Geometry check sheet. Reference: the model listing, model coordinates, mm. A direction names the side the tool comes from. Give positions to 0.01 mm unless a question says otherwise; leave off trailing zeros. Loops run counter-clockwise (first coordinate to the right, second up) from the corner with the lowest first, then second, coordinate; pieces in that order, holes last. Notation, with made-up numbers: (65, 88.5) -> (96, 88.5) arc R17 cw to (96, 100.5) -> close; hole circle Ø5 at (40, -15.75). An arc over 180 degrees is marked (long way). Answer in a Markdown table with one row per item. Add a question column.
```python
from build123d import *

# Parameters (mm, degrees)
CROQUIS1_W              = 72.136
CROQUIS1_H              = 25.4
SALIENTE_EXTRUIR1_DEPTH = 96.52
VACIADO1_T              = -3
CROQUIS2_W              = 2.032
CROQUIS2_H              = 17.272
SALIENTE_EXTRUIR3_DEPTH = 96.52
CROQUIS4_W              = 16.5
CROQUIS4_H              = 4
SALIENTE_EXTRUIR4_DEPTH = 4.5


with BuildPart() as part:
    # Croquis1 → Saliente-Extruir1 (new body)
    with BuildSketch(Plane.XY):
        with Locations((-36.068, 12.7)):
            Rectangle(CROQUIS1_W, CROQUIS1_H)
    extrude(amount=SALIENTE_EXTRUIR1_DEPTH)

    # Vaciado1
    vaciado1_openings = [part.faces().sort_by_distance(p)[0] for p in [
        (-36.068, 25.4, 48.26),
    ]]
    offset(amount=VACIADO1_T, openings=vaciado1_openings, kind=Kind.INTERSECTION)

    # Croquis2 → Saliente-Extruir3 (add)
    with BuildSketch(Plane(origin=(0, 0, 0), x_dir=(-1, 0, 0), z_dir=(0, 0, -1))):
        with Locations((-1.016, 12.7)):
            Rectangle(CROQUIS2_W, CROQUIS2_H)
        with Locations((73.152, 12.7)):
            Rectangle(CROQUIS2_W, CROQUIS2_H)
    extrude(amount=-SALIENTE_EXTRUIR3_DEPTH)

    # Croquis4 → Saliente-Extruir4 (add)
    with BuildSketch(Plane(origin=(0, 0, 0), x_dir=(-1, 0, 0), z_dir=(0, 0, -1))):
        with Locations((36.068, 3.262624702)):
            Rectangle(CROQUIS4_W, CROQUIS4_H)
    extrude(amount=SALIENTE_EXTRUIR4_DEPTH)


solid = part.part
```
1. Sectioned sample at D-D (y = 22.5). Enter the section's corners in (x, z).
2. Material ranges on L1, parallel to X at y = 11.5, z = 55; L2, parallel to Z at x = -30, y = 12.75; L3, parallel to X at y = 21.75, z = 85, recorded low to high. Write a range as from..to.
3. Sectioned sample at C-C (x = -9). Enter the section's corners in (y, z), plus the area to 3 significant figures.
4. Gauge pin test, flat ends, axial feed: pin 1 Ø1.3 at (x, z) = (-37, -2.5) entering from -Y; pin 2 Ø4.5 at (y, z) = (2.5, -3) entering from -X; pin 3 Ø2 at (y, z) = (23, 30.5) entering from -X. Record the tip position at first contact, or that the pin passes through.
5. Sectioned sample at B-B (z = 31.5). Enter the section's corners in (x, y), plus the area to 3 significant figures.
6. Sectioned sample at A-A (y = 13.25). Enter the section's corners in (x, z), plus the area to 3 significant figures.
7. Access from +Z, -Z, +X, -X, +Y, -Y to the whole of each face (thin tool, end or side, straight path). Record for faces 1 (the face through (-36, 5.263, -2)), 2 (the face through (1, 21.336, 48)), 3 (the face through (1, 4.064, 48)).
8. Release check for a two-part mould opening along X. For faces 4 (the face through (-36, 3, -4.5)), 5 (the face through (-37, 14, 93.52)), 6 (the face through (-72.136, 23, 48)) record: released by +X, released by -X, zero draft, split by the parting line, or undercut.
Response:
| question | item | result |
|---|---|---|
| 1 | outline | (-72.14, 0) -> (0, 0) -> (0, 96.52) -> (-72.14, 96.52) -> close; hole (-69.14, 3) -> (-3, 3) -> (-3, 93.52) -> (-69.14, 93.52) -> close |
| 2 | L1 | x = -74.17..-69.14, -3..2.03 |
| 2 | L2 | z = 0..3, 93.52..96.52 |
| 2 | L3 | x = -72.14..-69.14, -3..0 |
| 3 | outline | (0, 0) -> (25.4, 0) -> (25.4, 3) -> (3, 3) -> (3, 93.52) -> (25.4, 93.52) -> (25.4, 96.52) -> (0, 96.52) -> close |
| 3 | area | 424 mm2 |
| 4 | pin 1 | stops at y = 1.26 |
| 4 | pin 2 | stops at x = -44.32 |
| 4 | pin 3 | stops at x = -72.14 |
| 5 | outline | (-74.17, 4.06) -> (-72.14, 4.06) -> (-72.14, 0) -> (0, 0) -> (0, 4.06) -> (2.03, 4.06) -> (2.03, 21.34) -> (0, 21.34) -> (0, 25.4) -> (-3, 25.4) -> (-3, 3) -> (-69.14, 3) -> (-69.14, 25.4) -> (-72.14, 25.4) -> (-72.14, 21.34) -> (-74.17, 21.34) -> close |
| 5 | area | 421 mm2 |
| 6 | outline | (-74.17, 0) -> (2.03, 0) -> (2.03, 96.52) -> (-74.17, 96.52) -> close; hole (-69.14, 3) -> (-3, 3) -> (-3, 93.52) -> (-69.14, 93.52) -> close |
| 6 | area | 1,370 mm2 |
| 7 | face 1 | -Z, +X, -X, +Y |
| 7 | face 2 | +Z, -Z, +X, +Y |
| 7 | face 3 | +Z, -Z, +X, -Y |
| 8 | face 4 | zero draft |
| 8 | face 5 | undercut |
| 8 | face 6 | released by -X |
